Read the model definition and answer for the solid it produces. Units are mm, in the model's axes. Give positions to 0.01 mm unless a question says otherwise; leave off trailing zeros. Loops run counter-clockwise (first coordinate to the right, second up) from the corner with the lowest first, then second, coordinate; pieces in that order, holes last. Notation, with made-up numbers: (-21.5, 41.25) -> (20.5, 41.25) arc R28 cw to (20.5, 61.25) -> close; hole circle Ø3 at (69, -24). An arc over 180 degrees is marked (long way). Answer as CSV lines item,"result". Start each with the question number.
```python
from build123d import *

# Parameters (mm, degrees)
SKETCH_1_R          = 1.625
EXTRUDE_1_DEPTH     = 3
CHAMFER_1_SIZE      = 0.5
CUT_EXTRUDE_1_DEPTH = 10
CHAMFER_2_SIZE      = 0.5
EXTRUDE_2_DEPTH     = 3


with BuildPart() as part:
    # 草图1 → 凸台-拉伸1 (new body)
    with BuildSketch(Plane(origin=(-1.5, 0, 0), x_dir=(0, -1, 0), z_dir=(-1, 0, 0))):
        with BuildLine():
            Line((-4.409830069, -22.795084974), (5.590169942, -2.795084974))
            ThreePointArc((5.590169942, -2.795084974), (5.897676995, 2.068793383), (2.619113609, 5.674746153))
            Line((2.619113609, 5.674746153), (-29.880886391, 20.674746153))
            ThreePointArc((-29.880886391, 20.674746153), (-37.215506358, 19.102011676), (-37.757365472, 11.620265055))
            Line((-37.757365472, 11.620265055), (-15.257365483, -23.379734945))
            ThreePointArc((-15.257365483, -23.379734945), (-9.663631759, -26.240941948), (-4.409830069, -22.795084974))
        make_face()
        with Locations(Location((0, 0, 0), (0, 0, 270))):
            Circle(SKETCH_1_R, mode=Mode.SUBTRACT)
        with Locations(Location((-32.5, 15, 0), (0, 0, 270))):
            Circle(SKETCH_1_R, mode=Mode.SUBTRACT)
        with Locations(Location((-10.000000011, -20, 0), (0, 0, 270))):
            Circle(SKETCH_1_R, mode=Mode.SUBTRACT)
        with BuildLine():
            Line((-25.696229087, 9.501814319), (-12.177289309, -11.527647568))
            ThreePointArc((-12.177289309, -11.527647568), (-12.703025857, -13.946035685), (-15.121413973, -13.420299137))
            Line((-15.121413973, -13.420299137), (-28.640353751, 7.60916275))
            ThreePointArc((-28.640353751, 7.60916275), (-28.114617204, 10.027550867), (-25.696229087, 9.501814319))
        make_face(mode=Mode.SUBTRACT)
        with BuildLine():
            Line((-15.542003206, 7.113468289), (-6.078745362, -7.607155033))
            ThreePointArc((-6.078745362, -7.607155033), (-6.604481909, -10.025543149), (-9.022870026, -9.499806601))
            Line((-9.022870026, -9.499806601), (-18.48612787, 5.22081672))
            ThreePointArc((-18.48612787, 5.22081672), (-17.960391323, 7.639204836), (-15.542003206, 7.113468289))
        make_face(mode=Mode.SUBTRACT)
    extrude(amount=-EXTRUDE_1_DEPTH)

    # 倒角1
    chamfer_1_edges = [part.edges().sort_by_distance(p)[0] for p in [
        (1.5, -5.897676995, 2.068793383),
        (1.5, 13.630886391, 13.174746153),
        (1.5, 0, 1.625),
        (-1.5, 0, 1.625),
        (1.5, 32.5, 16.625),
        (1.5, 37.215506358, 19.102011676),
        (-1.5, 32.5, 16.625),
        (1.5, 10.000000011, -18.375),
        (1.5, 26.507365477, -5.879734945),
        (-1.5, 10.000000011, -18.375),
        (1.5, 28.114617204, 10.027550867),
        (1.5, 18.936759198, -1.012916624),
        (1.5, 12.703025857, -13.946035685),
        (1.5, 21.880883862, -2.905568193),
        (-1.5, 28.114617204, 10.027550867),
        (-1.5, 21.880883862, -2.905568193),
        (-1.5, 12.703025857, -13.946035685),
        (-1.5, 18.936759198, -1.012916624),
        (1.5, 17.960391323, 7.639204836),
        (1.5, 10.810374284, -0.246843372),
        (1.5, 6.604481909, -10.025543149),
        (1.5, 13.754498948, -2.139494941),
        (-1.5, 17.960391323, 7.639204836),
        (-1.5, 13.754498948, -2.139494941),
        (-1.5, 6.604481909, -10.025543149),
        (-1.5, 10.810374284, -0.246843372),
        (1.5, 9.663631759, -26.240941948),
        (-1.5, 26.507365477, -5.879734945),
        (-1.5, 37.215506358, 19.102011676),
        (-1.5, 13.630886391, 13.174746153),
        (-1.5, -5.897676995, 2.068793383),
        (-1.5, -0.590169937, -12.795084974),
        (-1.5, 9.663631759, -26.240941948),
        (1.5, -0.590169937, -12.795084974),
    ]]
    chamfer(chamfer_1_edges, length=CHAMFER_1_SIZE)

    # 草图2 → 切除-拉伸1 (cut)
    with BuildSketch(Plane(origin=(1.5, 0, 0), x_dir=(0, 0, -1), z_dir=(1, 0, 0))):
        with BuildLine():
            Line((-3.928015544, 10.805893754), (0.277876833, 8.102105799))
            ThreePointArc((0.277876833, 8.102105799), (0.803613381, 5.683717682), (-1.614774736, 5.157981135))
            Line((-1.614774736, 5.157981135), (-5.820667113, 7.86176909))
            ThreePointArc((-5.820667113, 7.86176909), (-6.346403661, 10.280157207), (-3.928015544, 10.805893754))
        make_face()
    extrude(amount=-CUT_EXTRUDE_1_DEPTH, mode=Mode.SUBTRACT)

    # 倒角2
    chamfer_2_edges = [part.edges().sort_by_distance(p)[0] for p in [
        (-1.5, 5.683717682, -0.803613381),
        (-1.5, 9.453999777, 1.825069356),
        (-1.5, 10.280157207, 6.346403661),
        (-1.5, 6.509875112, 3.717720925),
        (1.5, 9.453999777, 1.825069356),
        (1.5, 6.509875112, 3.717720925),
        (1.5, 5.683717682, -0.803613381),
        (1.5, 10.280157207, 6.346403661),
    ]]
    chamfer(chamfer_2_edges, length=CHAMFER_2_SIZE)

    # Sketch 3D_1 → 凸台-拉伸2 (add)
    with BuildSketch(Plane(origin=(1.5, 33.431032362, 9.779789625), x_dir=(0, -0.8679628670019027, -0.49662909852911097), z_dir=(1, 0, 0))):
        Polygon((0, 0), (27.366404933, 14.397799707), (33.391580963, 10.950327639), (36.801934048, 0), (32.111357291, -5.715828848), (26.004298505, -10.99963533), (16.146301167, -10.675777123), (2.885850361, -3.94968319), align=None)
    extrude(amount=-EXTRUDE_2_DEPTH)


solid = part.part
```
(1) Find section C-C on y = 0. Write down the section's boundary in (x, z) (3 decimals), then the cut area to 3 significant figures.
(2) Find the intervals of material crossed by line 1 along Y through (x, z) = (-0.3, 15) (3 decimals); line 2 along Y through (x, z) = (0.3, -20) (3 decimals); line 3 along Z through (x, y) = (-0.05, 32.5) (3 decimals), in increasing order. Write a range as from..to.
(3) Find section D-D on y = 22.5. Write down the section's boundary in (x, z), then the cut area to 3 significant figures.
(4) The mould has two halves that part along Y. Classify faces 1 (the face through (-0.01, 9.51, -21.55)), 2 (the face through (-1.365, 9.77, -25.881)), 3 (the face through (-0.01, -5.92, 2)): pulls with the +Y half, pulls with the -Y half, needs draft (parallel to the pull), parting line crosses it, or undercut.
(5) Each of these flat-tipped pins is pushed along its axis until it touches: P1, Ø2.5, axis at y = 0, z = 0, coming from the -X side; P2, Ø1.5, axis at x = 0, y = 22, coming from the -Z side; P3, Ø1.5, axis at x = 0.5, y = 30, coming from the +Z side; P4, Ø3, axis at y = 1, z = -18.5, coming from the -X side. Where does it stop, or does it pass through?
(6) Find section B-B on z = 0. Write down the section's boundary in (x, y) (3 decimals).
(7) Find section A-A on x = 0. Write down the section's boundary in (y, z) (3 decimals), then the cut area to 3 significant figures.
Answer block:
1,outline,"(-1.5, -12.857) -> (-1, -13.975) -> (1, -13.975) -> (1.5, -12.857) -> (1.5, -2.125) -> (1, -1.625) -> (-1, -1.625) -> (-1.5, -2.125) -> close; (-1.5, 2.125) -> (-1, 1.625) -> (1, 1.625) -> (1.5, 2.125) -> (1.5, 6.333) -> (1, 6.884) -> (-1, 6.884) -> (-1.5, 6.333) -> close"
1,area,"51.5 mm2"
2,line 1,"y = 17.586..30.875, 34.125..38.75"
2,line 2,"y = 3.012..8.375, 11.625..17.43"
2,line 3,"z = 3.442..13.375, 16.625..21.25"
3,outline,"(-1.5, -11.19) -> (-1, -12.11) -> (1, -12.11) -> (1.5, -11.19) -> (1.5, 16.72) -> (1, 17.27) -> (-1, 17.27) -> (-1.5, 16.72) -> close"
3,area,"87.4 mm2"
4,face 1,"undercut"
4,face 2,"parting line crosses it"
4,face 3,"pulls with the -Y half"
5,P1,"passes through"
5,P2,"stops at z = -14.06"
5,P3,"stops at z = 21"
5,P4,"stops at x = -1.37"
6,outline,"(-1.5, -5.75) -> (-1, -6.25) -> (1, -6.25) -> (1.5, -5.75) -> (1.5, -2.125) -> (1, -1.625) -> (-1, -1.625) -> (-1.5, -2.125) -> close; (-1.5, 2.125) -> (-1, 1.625) -> (1, 1.625) -> (1.5, 2.125) -> (1.5, 29.693) -> (1, 30.287) -> (-1, 30.287) -> (-1.5, 29.693) -> close"
7,outline,"(-5.59, -2.795) -> (4.41, -22.795) arc R6.25 ccw to (15.257, -23.38) -> (37.757, 11.62) arc R6.25 ccw to (29.881, 20.675) -> (-2.619, 5.675) arc R6.25 ccw to start; hole circle Ø3.25 at (0, 0); hole circle Ø3.25 at (10, -20); hole circle Ø3.25 at (32.5, 15)"
7,area,"1,120 mm2"
